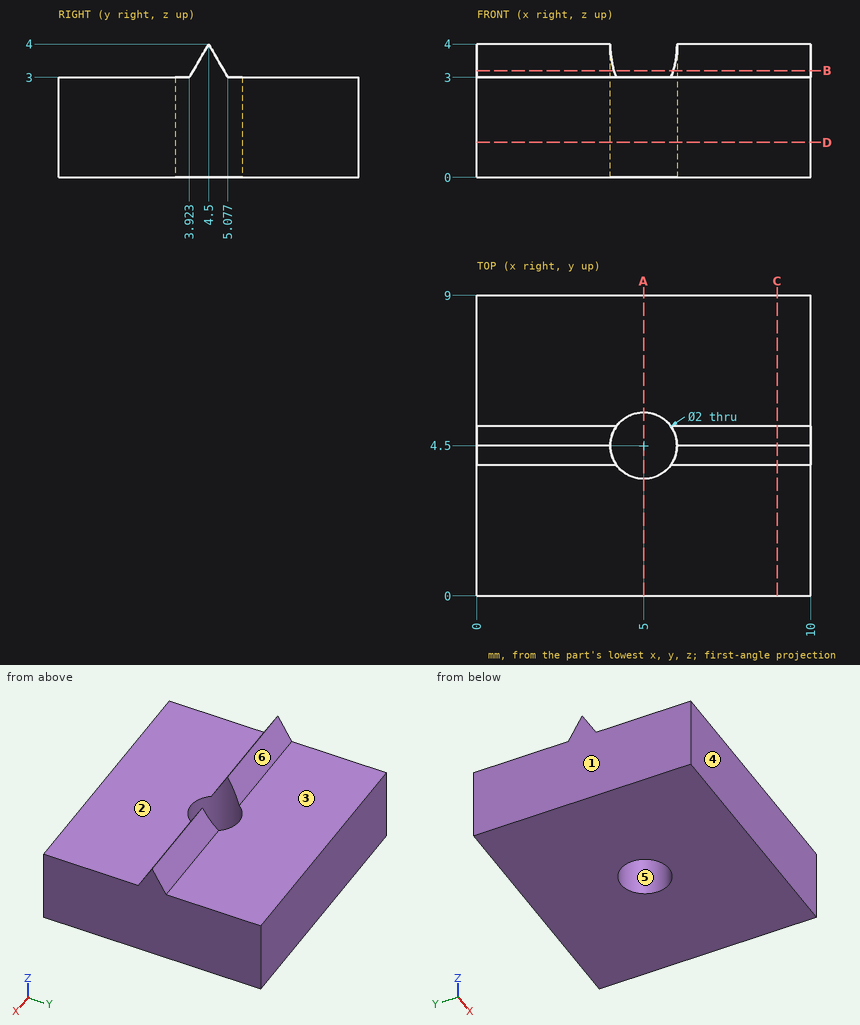
Source: three-view drawing plus pictorial views. Frame: mm from the lowest corner of the part. A direction names the side the tool comes from. Give positions to 0.01 mm unless a question says otherwise; leave off trailing zeros. Loops run counter-clockwise (first coordinate to the right, second up) from the corner with the lowest first, then second, coordinate; pieces in that order, holes last. Notation, with made-up numbers: M -17.5,25 L 30.5,25 A29 ccw 30.5,61 Z; hole C 22,28 d4. An arc over 180 degrees is marked long. Use CSV: the item, a comma, the result in double quotes.
(1) Pin query (flat end, axial travel): P1, Ø1, axis at x = 4, y = 6.5, coming from the -Z side; P2, Ø3, axis at x = 3.5, y = 2.5, coming from the +Z side (1 decimal); P3, Ø1.2, axis at x = 3.5, y = 8, coming from the +Z side. Return the tip coordinate at first contact, or that it passes through.
Outcome:
P1,"stops at z = 0"
P2,"stops at z = 3.1"
P3,"stops at z = 3"
(2) Section B-B, the plane z = 3.2. Return loops of the section in (x, y).
Outcome:
outline,"M 0,4.04 L 4.11,4.04 A1 cw 4.11,4.96 L 0,4.96 Z; M 5.89,4.04 L 10,4.04 L 10,4.96 L 5.89,4.96 A1 cw Z"
(3) Set-up query: the marked faces 1, 2 and 3. Return all of +Z, -Z, +X, -X, +Y, -Y with unobstructed straight access to the full face (end or side cutting, diameter ignored); none if empty.
Outcome:
face 1,"+Z, -Z, -X, +Y, -Y"
face 2,"+Z, +X, -X, -Y"
face 3,"+Z, +X, -X, +Y"
(4) Section D-D, the plane z = 1.05. Return loops of the section in (x, y).
Outcome:
outline,"M 0,0 L 10,0 L 10,9 L 0,9 Z; hole C 5,4.5 d2"
(5) Section A-A, the plane x = 5. Return loops of the section in (y, z), plus the area to 3 significant figures.
Outcome:
outline,"M 0,0 L 3.5,0 L 3.5,3 L 0,3 Z; M 5.5,0 L 9,0 L 9,3 L 5.5,3 Z"
area,"21.0 mm²"
(6) Section C-C, the plane x = 9. Return loops of the section in (y, z).
Outcome:
outline,"M 0,0 L 9,0 L 9,3 L 5.08,3 L 4.5,4 L 3.92,3 L 0,3 Z"
(7) Pull-direction query (Y, two-part tool) for the marked faces 4, 5 and 6; classes: pulls with the +Y half, pulls with the -Y half, needs draft (parallel to the pull), parting line crosses it, or undercut.
Outcome:
face 4,"pulls with the -Y half"
face 5,"undercut"
face 6,"pulls with the +Y half"
(8) Material intervals for L1, parallel to Y at x = 5, z = 1.35; L2, parallel to X at y = 4.5, z = 1.75; L3, parallel to Z at x = 6, y = 3, sorted ascending. Write a range as [from, to].
Outcome:
L1,"y = [0, 3.5], [5.5, 9]"
L2,"x = [0, 4], [6, 10]"
L3,"z = [0, 3]"
